from build123d import *

# Parameters (mm, degrees)
BOSS_EXTRUDE1_DEPTH                      = 8
F_3_9_3_9_DIAMETER_HOLE1_D               = 3.9
F_3_9_3_9_DIAMETER_HOLE1_DEPTH           = 6
F_3_9_3_9_DIAMETER_HOLE1_TIP             = 1.95
F_3_9_3_9_DIAMETER_HOLE1_ON_FACE_2_D     = 3.9
F_3_9_3_9_DIAMETER_HOLE1_ON_FACE_2_DEPTH = 6
F_3_9_3_9_DIAMETER_HOLE1_ON_FACE_2_TIP   = 1.95
F_3_9_3_9_DIAMETER_HOLE1_ON_FACE_3_D     = 3.9
F_3_9_3_9_DIAMETER_HOLE1_ON_FACE_3_DEPTH = 6
F_3_9_3_9_DIAMETER_HOLE1_ON_FACE_3_TIP   = 1.95
F_3_4_START                              = -8
F_3_4_3_4_DIAMETER_HOLE1_OUTLINE_R       = 1.7
F_3_4_3_4_DIAMETER_HOLE1_DEPTH           = 1.7500001
F_3_4_3_4_DIAMETER_HOLE1_2_OUTLINE_R     = 1.7
F_3_4_3_4_DIAMETER_HOLE1_2_DEPTH         = 1.7500001
F_3_4_3_4_DIAMETER_HOLE1_3_OUTLINE_R     = 1.7
F_3_4_3_4_DIAMETER_HOLE1_3_DEPTH         = 1.7500001
FILLET1_R                                = 0.5


# Read off the part's stored shape, not the designer's step: Ø3.4 (3.4) Diameter Hole1
with BuildPart() as part:
    # Sketch1 → Boss-Extrude1 (new body)
    with BuildSketch(Plane.XY):
        Polygon((0, 0), (0, 8), (-8, 8), (-8, -8), (8, -8), (8, 0), align=None)
    extrude(amount=BOSS_EXTRUDE1_DEPTH)

    # Ø3.9 (3.9) Diameter Hole1
    with Locations(Plane(origin=(-4, -4, 8), x_dir=(1, 0, 0), z_dir=(0, 0, 1))):
        with Locations((0, 0)):
            Hole(F_3_9_3_9_DIAMETER_HOLE1_D / 2, depth=F_3_9_3_9_DIAMETER_HOLE1_DEPTH)
            with Locations((0, 0, -(F_3_9_3_9_DIAMETER_HOLE1_DEPTH + F_3_9_3_9_DIAMETER_HOLE1_TIP / 2))):  # 90° drill point
                Cone(0, F_3_9_3_9_DIAMETER_HOLE1_D / 2, F_3_9_3_9_DIAMETER_HOLE1_TIP, mode=Mode.SUBTRACT)

    # Ø3.9 (3.9) Diameter Hole1 on face 2
    with Locations(Plane(origin=(0, 4, 4), x_dir=(0, 0, 1), z_dir=(1, 0, 0))):
        with Locations((0, 0)):
            Hole(F_3_9_3_9_DIAMETER_HOLE1_ON_FACE_2_D / 2, depth=F_3_9_3_9_DIAMETER_HOLE1_ON_FACE_2_DEPTH)
            with Locations((0, 0, -(F_3_9_3_9_DIAMETER_HOLE1_ON_FACE_2_DEPTH + F_3_9_3_9_DIAMETER_HOLE1_ON_FACE_2_TIP / 2))):  # 90° drill point
                Cone(0, F_3_9_3_9_DIAMETER_HOLE1_ON_FACE_2_D / 2, F_3_9_3_9_DIAMETER_HOLE1_ON_FACE_2_TIP, mode=Mode.SUBTRACT)

    # Ø3.9 (3.9) Diameter Hole1 on face 3
    with Locations(Plane(origin=(4, 0, 4), x_dir=(0, 0, 1), z_dir=(0, 1, 0))):
        with Locations((0, 0)):
            Hole(F_3_9_3_9_DIAMETER_HOLE1_ON_FACE_3_D / 2, depth=F_3_9_3_9_DIAMETER_HOLE1_ON_FACE_3_DEPTH)
            with Locations((0, 0, -(F_3_9_3_9_DIAMETER_HOLE1_ON_FACE_3_DEPTH + F_3_9_3_9_DIAMETER_HOLE1_ON_FACE_3_TIP / 2))):  # 90° drill point
                Cone(0, F_3_9_3_9_DIAMETER_HOLE1_ON_FACE_3_D / 2, F_3_9_3_9_DIAMETER_HOLE1_ON_FACE_3_TIP, mode=Mode.SUBTRACT)

    # Ø3.4 (3.4) Diameter Hole1 outline → Ø3.4 (3.4) Diameter Hole1 (cut)
    with BuildSketch(Plane(origin=(0, 0, 0), x_dir=(1, 0, 0), z_dir=(0, 1, 0)).offset(F_3_4_START)):
        with Locations((4, -4)):
            Circle(F_3_4_3_4_DIAMETER_HOLE1_OUTLINE_R)
    extrude(amount=F_3_4_3_4_DIAMETER_HOLE1_DEPTH, mode=Mode.SUBTRACT)

    # 3.4 _3.4_ Diameter Hole1 2 outline → 3.4 _3.4_ Diameter Hole1 2 (cut)
    with BuildSketch(Plane.YZ.offset(F_3_4_START)):
        with Locations((4, 4)):
            Circle(F_3_4_3_4_DIAMETER_HOLE1_2_OUTLINE_R)
    extrude(amount=F_3_4_3_4_DIAMETER_HOLE1_2_DEPTH, mode=Mode.SUBTRACT)

    # 3.4 _3.4_ Diameter Hole1 3 outline → 3.4 _3.4_ Diameter Hole1 3 (cut)
    with BuildSketch(Plane.XY):
        with Locations((-4, -4)):
            Circle(F_3_4_3_4_DIAMETER_HOLE1_3_OUTLINE_R)
    extrude(amount=F_3_4_3_4_DIAMETER_HOLE1_3_DEPTH, mode=Mode.SUBTRACT)

    # Fillet1
    fillet1_edges = [part.edges().sort_by_distance(p)[0] for p in [
        (8, 0, 4),
        (8, -8, 4),
        (-8, -8, 4),
        (-8, 8, 4),
        (0, 8, 4),
        (0, 0, 4),
        (-4, 8, 8),
        (-8, 0, 8),
        (0, -8, 8),
        (8, -4, 8),
        (4, 0, 8),
        (8, -4, 0),
        (0, -8, 0),
        (-8, 0, 0),
        (-4, 8, 0),
        (0, 4, 0),
        (4, 0, 0),
        (0, 4, 8),
    ]]
    fillet(fillet1_edges, radius=FILLET1_R)


solid = part.part
Design review of the part built by this model. Coordinates are the model's own, in mm. A direction names the side the tool comes from. Round coordinates to 2 decimals unless told otherwise and drop trailing zeros. Loops run counter-clockwise (first coordinate to the right, second up) from the corner with the lowest first, then second, coordinate; pieces in that order, holes last. Notation, with made-up numbers: (-16, 88) - (-9, 88) arc R6 ccw to (-9, 94) - close; hole circle Ø8 at (81, -3.5). An arc over 180 degrees is marked (long way). One line per question, with ' | ' between items.
1. We need section A-A, the plane z = 4. State how many separate pieces and enclosed holes the cut face has, and give its area (3 significant figures).
Results are:
separate pieces: 3 | enclosed holes: 1 | area: 119 mm²
2. For faces 1 (the face through (2.813, -3.042, 5.547)), 2 (the face through (-3.042, 5.187, 5.547)), 3 (the face through (-2.453, -5.187, 4.958)), 4 (the face through (0, 2, 6)), 5 (the face through (-2, -2, 0)), list the 3-axis set-ups (+Z, -Z, +X, -X, +Y, -Y) from which the entire face can be reached by the end or side of a thin tool; tool diameter is ignored.
Results are:
face 1: +Y | face 2: +X | face 3: +Z | face 4: +Z, -Z, +X, +Y | face 5: -Z, +X, -X, +Y, -Y
3. We need section D-D, the plane x = 4. State the section outline as (y, z) points, and give its area (3 significant figures).
Results are:
outline: (-8, 0.5) arc R0.5 ccw to (-7.5, 0) - (-0.5, 0) arc R0.5 ccw to (0, 0.5) - (0, 2.05) - (-6, 2.05) - (-6.25, 2.3) - (-8, 2.3) - close; (-8, 5.7) - (-6.25, 5.7) - (-6, 5.95) - (0, 5.95) - (0, 7.5) arc R0.5 ccw to (-0.5, 8) - (-7.5, 8) arc R0.5 ccw to (-8, 7.5) - close | area: 33.5 mm²
4. Clearance check with flat-ended pins moving along their axes: P1, Ø3.5, axis at y = 3, z = 2.5, coming from the +X side; P2, Ø2, axis at x = 5, z = 5.5, coming from the +Y side. State where each tip first meets the part, or that it passes through.
Results are:
P1: stops at x = 0 | P2: stops at y = 0
5. For L1, parallel to X at y = -1.45, z = 4; L2, parallel to X at y = -5.5, z = 5.25; L3, parallel to Y at x = -4, z = 5.75, list the stretches that pass through material, from the lowest coordinate up. Write a range as [from, to].
Results are:
L1: x = [-8, 2.05], [5.95, 8] | L2: x = [-8, -5.25], [-2.75, 2.5], [5.5, 8] | L3: y = [-8, -5.95], [-2.05, 3.14], [4.86, 8]
6. Draft analysis for pull direction Y (two halves, no side actions). For faces 6 (the face through (6, 0, 6)), 7 (the face through (-2, -2, 8)), 8 (the face through (-7.14, 5.57, 3.35)), state which applies: released by +Y, released by -Y, zero draft, split by the parting line, or undercut.
Results are:
face 6: released by +Y | face 7: zero draft | face 8: undercut
7. We need section B-B, the plane y = -4. State the section outline as (x, z) points.
Results are:
outline: (-8, 0.5) arc R0.5 ccw to (-7.5, 0) - (-5.7, 0) - (-5.7, 1.75) - (-5.95, 2) - (-5.95, 8) - (-7.5, 8) arc R0.5 ccw to (-8, 7.5) - close; (-2.3, 0) - (7.5, 0) arc R0.5 ccw to (8, 0.5) - (8, 7.5) arc R0.5 ccw to (7.5, 8) - (-2.05, 8) - (-2.05, 2) - (-2.3, 1.75) - close; hole circle Ø3.9 at (4, 4)
